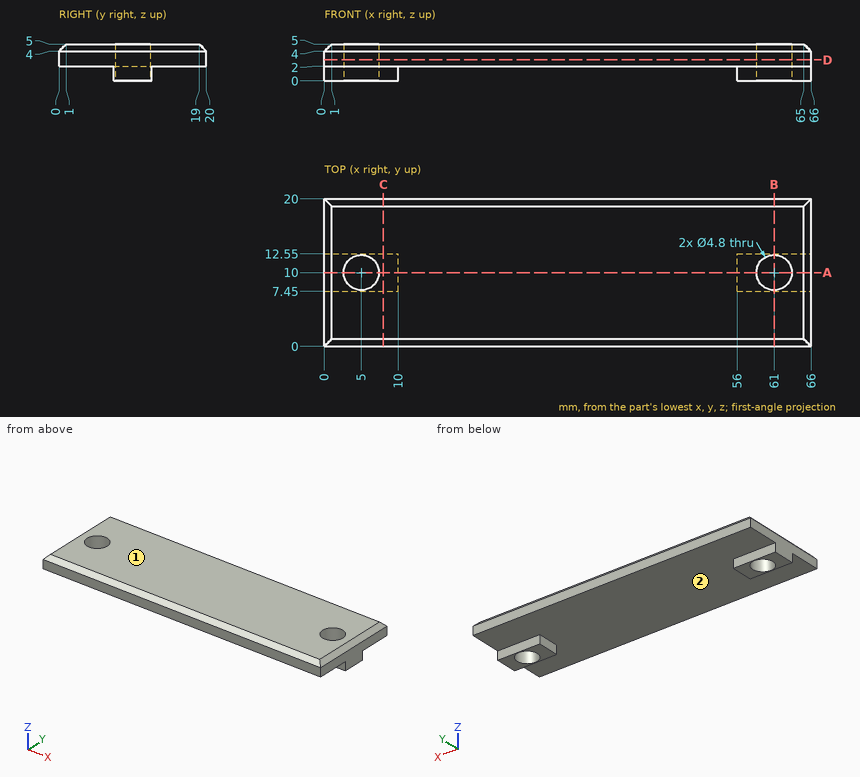
Check sheet for the drawn part. Datum: minimum x, y, z corner. Units: mm. Round coordinates to 2 decimals unless told otherwise and drop trailing zeros. Write each loop counter-clockwise with the first axis right and the second up, starting at its lowest first coordinate (ties: lowest second). Pieces come first, ordered by that corner, then holes. Notation, with made-up numbers: (-26, 7.25) -> (-4, 7.25) arc R18 ccw to (-4, 21.25) -> close; hole circle Ø1 at (-13.75, -8.75). An arc over 180 degrees is marked (long way). One line per item, written item: value. Start each with the question number.
(1) Cross-section at C-C, the plane x = 8. Record the cut outline in (y, z), and give its area (3 significant figures).
(2) Cross-section at A-A, the plane y = 10. Record the cut outline in (x, z).
(3) Go/stop test with flat-tipped pins: pin 1 Ø3 at (x, y) = (26.5, 12) entering from -Z; pin 2 Ø2 at (x, z) = (59.5, 0.5) entering from -Y; pin 3 Ø1 at (x, z) = (5.5, 0.5) entering from +Y. Record where each tip stops, or that it passes through.
(4) Cross-section at B-B, the plane x = 61. Record the cut outline in (y, z), and give its area (3 significant figures).
(5) Draft check along X on the marked faces 1 and 2. Enter one of: +X half, -X half, draft (parallel to the pull), parting line (faces both ways), or undercut.
(6) Scan lines: line 1 (Y direction, x = 5, z = 2.75); line 2 (Z direction, x = 50, y = 1.5); line 3 (Y direction, x = 60, z = 3.9). Record each from-to range of solid material in increasing order. Write a range as [from, to].
(7) Cross-section at D-D, the plane z = 2.85. Record the cut outline in (x, y).
Answer:
1. outline: (0, 2) -> (7.45, 2) -> (7.45, 0) -> (12.55, 0) -> (12.55, 2) -> (20, 2) -> (20, 4) -> (19, 5) -> (1, 5) -> (0, 4) -> close
1. area: 69.2 mm²
2. outline: (0, 0) -> (2.6, 0) -> (2.6, 5) -> (1, 5) -> (0, 4) -> close; (7.4, 0) -> (10, 0) -> (10, 2) -> (56, 2) -> (56, 0) -> (58.6, 0) -> (58.6, 5) -> (7.4, 5) -> close; (63.4, 0) -> (66, 0) -> (66, 4) -> (65, 5) -> (63.4, 5) -> close
3. pin 1: z = 2
3. pin 2: y = 7.45
3. pin 3: y = 12.55
4. outline: (0, 2) -> (7.45, 2) -> (7.45, 0) -> (7.6, 0) -> (7.6, 5) -> (1, 5) -> (0, 4) -> close; (12.4, 0) -> (12.55, 0) -> (12.55, 2) -> (20, 2) -> (20, 4) -> (19, 5) -> (12.4, 5) -> close
4. area: 45.2 mm²
5. face 1: draft
5. face 2: undercut
6. line 1: [0, 7.6], [12.4, 20]
6. line 2: [2, 5]
6. line 3: [0, 7.82], [12.18, 20]
7. outline: (0, 0) -> (66, 0) -> (66, 20) -> (0, 20) -> close; hole circle Ø4.8 at (5, 10); hole circle Ø4.8 at (61, 10)
